Answer from the drawing. Dimensions are ordinates in mm from the lowest x, y and z of the part. Round coordinates to 2 decimals unless told otherwise and drop trailing zeros. Loops run counter-clockwise (first coordinate to the right, second up) from the corner with the lowest first, then second, coordinate; pieces in that order, holes last. Notation, with made-up numbers: M 49.25,-25.75 L 71.25,-25.75 A30 cw 71.25,3.25 Z; hole C -20.5,-25 d7. An arc over 180 degrees is marked long. Answer as a JSON object with one key per item and string values.
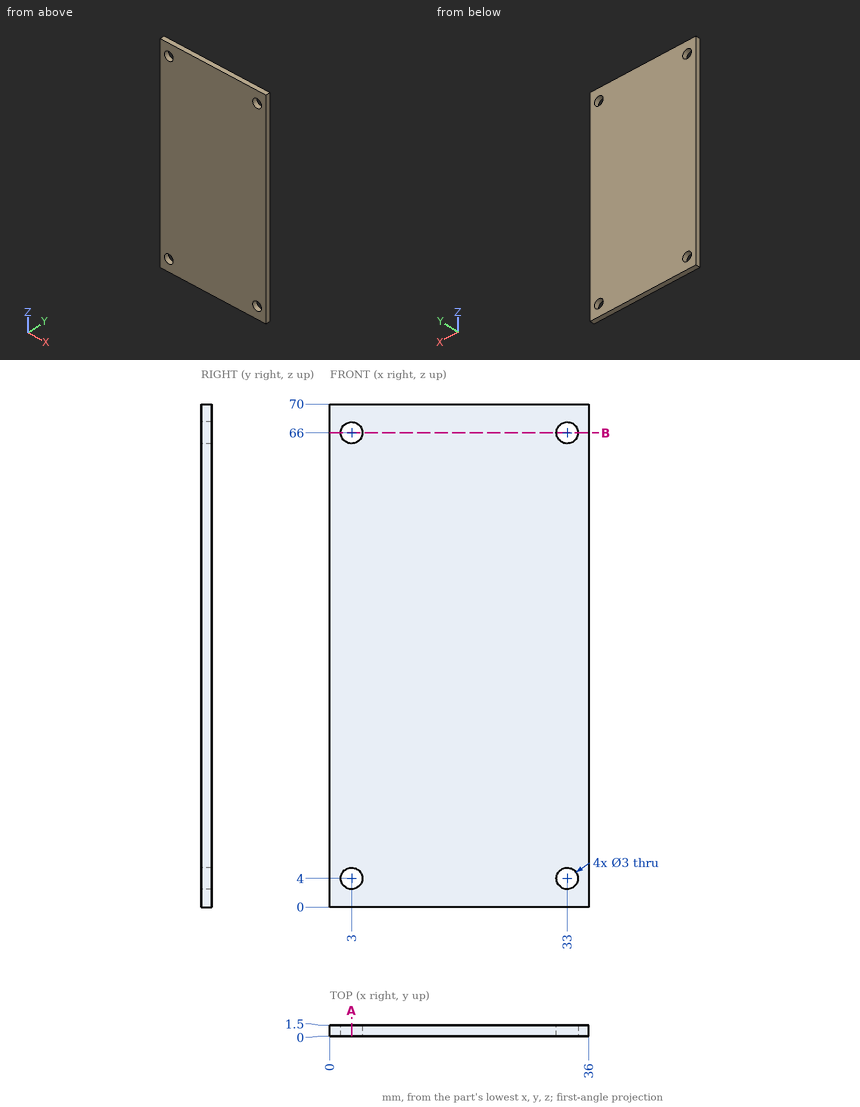
Item 1: The part is cut by section B-B (z = 66). Give the vertices of the cut face in (x, y).
Values follow:
{"outline": "M 0,0 L 1.5,0 L 1.5,1.5 L 0,1.5 Z; M 4.5,0 L 31.5,0 L 31.5,1.5 L 4.5,1.5 Z; M 34.5,0 L 36,0 L 36,1.5 L 34.5,1.5 Z"}
Item 2: Straight lines are drawn through the part: line 1 (X direction, y = 0.85, z = 66); line 2 (Z direction, x = 3, y = 0.8); line 3 (Z direction, x = 2.5, y = 1.35). For each, find the intervals that lie inside material, in ascending order.
Values follow:
{"line 1": "0 to 1.5, 4.5 to 31.5, 34.5 to 36", "line 2": "0 to 2.5, 5.5 to 64.5, 67.5 to 70", "line 3": "0 to 2.59, 5.41 to 64.59, 67.41 to 70"}
Item 3: The part is cut by section A-A (x = 3). Give the vertices of the cut face in (y, z), then the cut area to 3 significant figures.
Values follow:
{"outline": "M 0,0 L 1.5,0 L 1.5,2.5 L 0,2.5 Z; M 0,5.5 L 1.5,5.5 L 1.5,64.5 L 0,64.5 Z; M 0,67.5 L 1.5,67.5 L 1.5,70 L 0,70 Z", "area": "96.0 mm^2"}
